Read the model definition and answer for the solid it produces. Units are mm, in the model's axes. Face numbers are marked on the shaded views. A direction names the side the tool comes from. Give positions to 0.01 mm unless a question says otherwise; leave off trailing zeros. Order: outer loops, then holes, each group sorted by start corner. A loop starts at its lowest first (then second) coordinate and runs counter-clockwise, first axis right, second up. Notation, with made-up numbers: (37.25, 87.5) - (74.25, 87.5) arc R21 ccw to (74.25, 120.5) - close; hole circle Ø5 at (1.5, -12). An arc over 180 degrees is marked (long way). Use a Markdown table: item, result. Add a question column.
1. A cutting plane is placed at D-D on x = 30.5. Determine the outline of the cut face in (y, z).
2. A cutting plane is placed at A-A on x = 44.45. Determine the outline of the cut face in (y, z), and give its area (3 significant figures).
3. A cutting plane is placed at B-B on y = 38.1. Determine the outline of the cut face in (x, z), and give its area (3 significant figures).
4. Which of the six approach directions +Z, -Z, +X, -X, +Y, -Y give full straight-line access (tool end or side, diameter ignored) to the marked faces 1 and 2?
5. Flat-ended cylindrical pins translate along their axes: P1, Ø8, axis at x = 50.99, y = 38.1, coming from the -Z side; P2, Ø13.5, axis at x = 34.5, z = -34.5, coming from the +Y side. Find the tip coordinate at first contact, or state that the pin passes through.
6. A cutting plane is placed at C-C on z = -19.05. Determine the outline of the cut face in (x, y).
7. Consider L1, parallel to X at y = 38, z = -3; L2, parallel to X at y = 3.75, z = -19.05; L3, parallel to Y at x = 5, z = -5. Determine where each line is inside the solid, lowest interval first.
```python
from build123d import *

# Parameters (mm, degrees)
BOSS_EXTRUDE1_DEPTH = 57.15
SKETCH3_R           = 2.4892
CUT_EXTRUDE1_DEPTH  = 92.800885072
SKETCH4_R           = 3.3782
CUT_EXTRUDE2_DEPTH  = 89.44526556


with BuildPart() as part:
    # Sketch1 → Boss-Extrude1 (new body)
    with BuildSketch(Plane(origin=(0, 0, 0), x_dir=(0, 0, -1), z_dir=(1, 0, 0))):
        Polygon((0, 0), (0, 50.8), (6.35, 50.8), (6.35, 6.35), (50.8, 6.35), (50.8, 0), align=None)
    extrude(amount=BOSS_EXTRUDE1_DEPTH)

    # Sketch3 → Cut-Extrude1 (cut, through all)
    with BuildSketch(Plane.XY):
        with Locations((6.1595, 38.1)):
            Circle(SKETCH3_R)
        with Locations((50.9905, 38.1)):
            Circle(SKETCH3_R)
        with Locations((50.9905, 12.7)):
            Circle(SKETCH3_R)
        with Locations((6.1595, 12.7)):
            Circle(SKETCH3_R)
    extrude(amount=-CUT_EXTRUDE1_DEPTH, mode=Mode.SUBTRACT)

    # Sketch4 → Cut-Extrude2 (cut, through all)
    with BuildSketch(Plane(origin=(0, 6.35, 0), x_dir=(1, 0, 0), z_dir=(0, 1, 0))):
        with Locations(Location((12.7, 19.05, 0), (0, 0, 270))):
            Circle(SKETCH4_R)
        with Locations(Location((12.7, 44.45, 0), (0, 0, 270))):
            Circle(SKETCH4_R)
        with Locations(Location((44.45, 44.45, 0), (0, 0, 270))):
            Circle(SKETCH4_R)
        with Locations(Location((44.45, 19.05, 0), (0, 0, 270))):
            Circle(SKETCH4_R)
    extrude(amount=-CUT_EXTRUDE2_DEPTH, mode=Mode.SUBTRACT)


solid = part.part
```
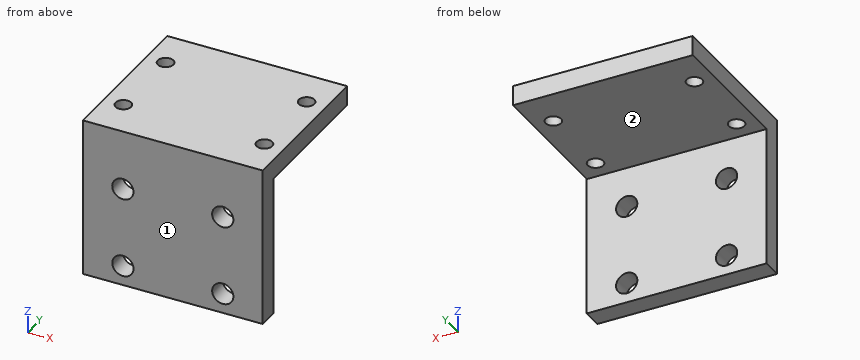
Output values:
| question | item | result |
|---|---|---|
| 1 | outline | (0, -50.8) - (6.35, -50.8) - (6.35, -6.35) - (50.8, -6.35) - (50.8, 0) - (0, 0) - close |
| 2 | outline | (0, -50.8) - (6.35, -50.8) - (6.35, -47.83) - (0, -47.83) - close; (0, -41.07) - (6.35, -41.07) - (6.35, -22.43) - (0, -22.43) - close; (0, -15.67) - (6.35, -15.67) - (6.35, -6.35) - (50.8, -6.35) - (50.8, 0) - (0, 0) - close |
| 2 | area | 519 mm² |
| 3 | outline | (0, -6.35) - (3.67, -6.35) - (3.67, 0) - (0, 0) - close; (8.65, -6.35) - (48.5, -6.35) - (48.5, 0) - (8.65, 0) - close; (53.48, -6.35) - (57.15, -6.35) - (57.15, 0) - (53.48, 0) - close |
| 3 | area | 300 mm² |
| 4 | face 1 | +Z, -Z, +X, -X, -Y |
| 4 | face 2 | -Z, +X, -X, +Y |
| 5 | P1 | z = -6.35 |
| 5 | P2 | y = 6.35 |
| 6 | outline | (0, 0) - (9.32, 0) - (9.32, 6.35) - (0, 6.35) - close; (16.08, 0) - (41.07, 0) - (41.07, 6.35) - (16.08, 6.35) - close; (47.83, 0) - (57.15, 0) - (57.15, 6.35) - (47.83, 6.35) - close |
| 7 | L1 | 0 to 3.67, 8.65 to 48.5, 53.48 to 57.15 |
| 7 | L2 | 0 to 9.32, 16.08 to 41.07, 47.83 to 57.15 |
| 7 | L3 | 0 to 10.5, 14.9 to 35.9, 40.3 to 50.8 |
